```python
from build123d import *

# Parameters (mm, degrees)
CROQUIS1_W              = 56.4
CROQUIS1_H              = 56.4
SALIENTE_EXTRUIR1_DEPTH = 49
CROQUIS2_R              = 19
SALIENTE_EXTRUIR2_DEPTH = 1.6
CROQUIS3_R              = 3.175
SALIENTE_EXTRUIR3_DEPTH = 22
CROQUIS4_R              = 2.5
CORTAR_EXTRUIR1_DEPTH   = 64.178160784
CROQUIS5_W              = 9
CROQUIS5_H              = 9
CORTAR_EXTRUIR2_DEPTH   = 44
REDONDEO1_R             = 4
REDONDEO2_R             = 2


with BuildPart() as part:
    # Croquis1 → Saliente-Extruir1 (new body)
    with BuildSketch(Plane.XY):
        Rectangle(CROQUIS1_W, CROQUIS1_H)
    extrude(amount=SALIENTE_EXTRUIR1_DEPTH)

    # Croquis2 → Saliente-Extruir2 (add)
    with BuildSketch(Plane.XY.offset(49)):
        Circle(CROQUIS2_R)
    extrude(amount=SALIENTE_EXTRUIR2_DEPTH)

    # Croquis3 → Saliente-Extruir3 (add)
    with BuildSketch(Plane.XY.offset(50.6)):
        Circle(CROQUIS3_R)
    extrude(amount=SALIENTE_EXTRUIR3_DEPTH)

    # Croquis4 → Cortar-Extruir1 (cut, through all)
    with BuildSketch(Plane.XY.offset(49)):
        with Locations((23.55, 23.55)):
            Circle(CROQUIS4_R)
        with Locations((-23.55, 23.55)):
            Circle(CROQUIS4_R)
        with Locations((-23.55, -23.55)):
            Circle(CROQUIS4_R)
        with Locations((23.55, -23.55)):
            Circle(CROQUIS4_R)
    extrude(amount=-CORTAR_EXTRUIR1_DEPTH, mode=Mode.SUBTRACT)

    # Croquis5 → Cortar-Extruir2 (cut)
    with BuildSketch(Plane(origin=(0, 0, 0), x_dir=(-1, 0, 0), z_dir=(0, 0, -1))):
        with Locations((-23.7, 23.7)):
            Rectangle(CROQUIS5_W, CROQUIS5_H)
        with Locations((23.7, 23.7)):
            Rectangle(CROQUIS5_W, CROQUIS5_H)
        with Locations((23.7, -23.7)):
            Rectangle(CROQUIS5_W, CROQUIS5_H)
        with Locations((-23.7, -23.7)):
            Rectangle(CROQUIS5_W, CROQUIS5_H)
    extrude(amount=-CORTAR_EXTRUIR2_DEPTH, mode=Mode.SUBTRACT)

    # Redondeo1
    redondeo1_edges = [part.edges().sort_by_distance(p)[0] for p in [
        (28.2, -28.2, 46.5),
        (-28.2, -28.2, 46.5),
        (-28.2, 28.2, 46.5),
        (28.2, 28.2, 46.5),
    ]]
    fillet(redondeo1_edges, radius=REDONDEO1_R)

    # Redondeo2
    redondeo2_edges = [part.edges().sort_by_distance(p)[0] for p in [
        (28.2, 19.2, 22),
        (19.2, 28.2, 22),
        (19.2, 19.2, 22),
        (-28.2, 19.2, 22),
        (-19.2, 19.2, 22),
        (-19.2, 28.2, 22),
        (-28.2, -19.2, 22),
        (-19.2, -28.2, 22),
        (-19.2, -19.2, 22),
        (28.2, -19.2, 22),
        (19.2, -19.2, 22),
        (19.2, -28.2, 22),
    ]]
    fillet(redondeo2_edges, radius=REDONDEO2_R)


solid = part.part
```
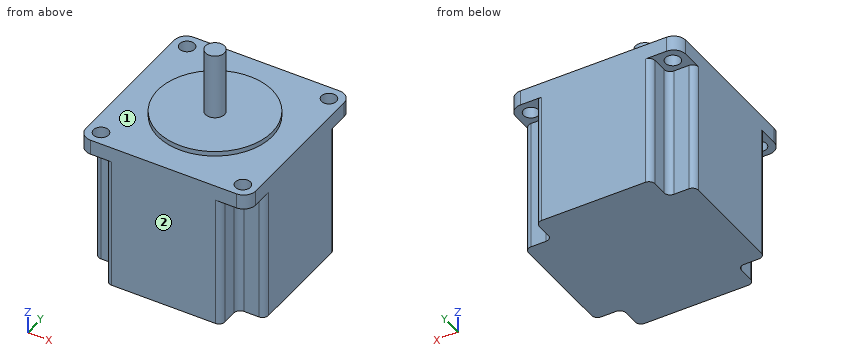
The listing builds one solid part. Answer for the finished solid, in the listing's coordinates (mm). Face numbers are marked on the shaded views. A direction names the side the tool comes from. Round coordinates to 2 decimals unless told otherwise and drop trailing zeros. Write each loop counter-clockwise with the first axis right and the second up, starting at its lowest first coordinate (ties: lowest second). Pieces come first, ordered by that corner, then holes. Notation, with made-up numbers: (-13.5, 28.5) -> (2.5, 28.5) arc R10 cw to (2.5, 37.5) -> close; hole circle Ø5 at (68.25, 68.25). An arc over 180 degrees is marked (long way). Answer as a JSON object with one key per item and string values. Group by question number.
Q1. Straight lines are drawn through the part: line 1 along Y through (x, z) = (23.55, 47.8); line 2 along Z through (x, y) = (-20.5, -22.5); line 3 along Z through (x, y) = (2.5, -13.5). For each, find the intervals that lie inside material, in ascending order.
Q2. Each of these flat-tipped pins is pushed along its axis until it touches: pin 1 Ø5 at (x, y) = (-5.5, 5.5) entering from +Z; pin 2 Ø4 at (y, z) = (-22.5, 30.5) entering from +X; pin 3 Ø3.5 at (x, y) = (21, 22) entering from -Z; pin 4 Ø4 at (x, y) = (23.55, 23.55) entering from +Z. Where does it stop, or does it pass through?
Q3. Section D-D (x = 7) is taken. Write down the section's boundary in (y, z).
Q4. Section A-A (y = 0) is taken. Write down the section's boundary in (x, z) (3 decimals).
Q5. Section B-B (z = 32.5) is taken. Write down the section's boundary in (x, y).
Q6. Which of the six approach directions +Z, -Z, +X, -X, +Y, -Y give full straight-line access (tool end or side, diameter ignored) to the marked faces 1 and 2?
Check values:
{
 "1": {"line 1": "-28.2 to -26.05, -21.05 to 21.05, 26.05 to 28.2", "line 2": "44 to 49", "line 3": "0 to 50.6"},
 "2": {"pin 1": "z = 50.6", "pin 2": "x = 19.33", "pin 3": "z = 44", "pin 4": "through"},
 "3": {"outline": "(-28.2, 0) -> (28.2, 0) -> (28.2, 49) -> (17.66, 49) -> (17.66, 50.6) -> (-17.66, 50.6) -> (-17.66, 49) -> (-28.2, 49) -> close"},
 "4": {"outline": "(-28.2, 0) -> (28.2, 0) -> (28.2, 49) -> (19, 49) -> (19, 50.6) -> (3.175, 50.6) -> (3.175, 72.6) -> (-3.175, 72.6) -> (-3.175, 50.6) -> (-19, 50.6) -> (-19, 49) -> (-28.2, 49) -> close"},
 "5": {"outline": "(-28.2, -17.2) arc R2 ccw to (-26.2, -19.2) -> (-21.2, -19.2) arc R2 cw to (-19.2, -21.2) -> (-19.2, -26.2) arc R2 ccw to (-17.2, -28.2) -> (17.2, -28.2) arc R2 ccw to (19.2, -26.2) -> (19.2, -21.2) arc R2 cw to (21.2, -19.2) -> (26.2, -19.2) arc R2 ccw to (28.2, -17.2) -> (28.2, 17.2) arc R2 ccw to (26.2, 19.2) -> (21.2, 19.2) arc R2 cw to (19.2, 21.2) -> (19.2, 26.2) arc R2 ccw to (17.2, 28.2) -> (-17.2, 28.2) arc R2 ccw to (-19.2, 26.2) -> (-19.2, 21.2) arc R2 cw to (-21.2, 19.2) -> (-26.2, 19.2) arc R2 ccw to (-28.2, 17.2) -> close"},
 "6": {"face 1": "+Z", "face 2": "+Z, -Z, +X, -X, -Y"}
}
